```python
from build123d import *

# Parameters (mm, degrees)
SKETCH_1_R               = 67.5
EXTRUDE_1_DEPTH          = 5
SKETCH_2_W               = 6
SKETCH_2_H               = 35
EXTRUDE_2_DEPTH          = 60
FILLET_1_R               = 17.5
SKETCH_3_R               = 16
CUT_EXTRUDE_1_DEPTH      = 5
CHAMFER_1_SIZE           = 1.640243073
CHAMFER_1_SIZE_2         = 0.8
SKETCH_4_R               = 15
CUT_EXTRUDE_2_DEPTH      = 121.188675061
SKETCH_6_W               = 2
SKETCH_6_H               = 6
CUT_EXTRUDE_3_DEPTH      = 121.817372977
SKETCH_8_R               = 1.6
CUT_EXTRUDE_5_DEPTH      = 6
CUT_EXTRUDE_START        = -2
CUT_EXTRUDE_8_DEPTH      = 2.2
SKETCH_11_W              = 25
SKETCH_11_H              = 10.5
EXTRUDE_4_DEPTH          = 7.3
EXTRUDE_5_DEPTH          = 2
FILLET_3_R               = 1
EXTRUDE_6_DEPTH          = 5
SKETCH_14_R              = 1.15
CUT_EXTRUDE_10_DEPTH     = 127.019830237
FILLET_2_R               = 0.5
SKETCH_15_R              = 2
CUT_EXTRUDE_11_DEPTH     = 10
SKETCH_16_W              = 56.328401117
SKETCH_16_H              = 65
CUT_EXTRUDE_12_DEPTH     = 2
SKETCH_17_W              = 112.249721604
SKETCH_17_H              = 30
CUT_EXTRUDE_13_DEPTH     = 113.749722891
SKETCH2_W                = 0.5
SKETCH2_H                = 16.5
BOSS_EXTRUDE1_DEPTH      = 6
BOSS_EXTRUDE2_DEPTH      = 0.5
BOSS_EXTRUDE2_DEPTH_BACK = 3
FILLET1_R                = 1
BOSS_EXTRUDE3_DEPTH      = 0.5
SKETCH5_OUTSIDE_W        = 173.686
SKETCH5_OUTSIDE_H        = 144.186
SKETCH5_OUTSIDE_R        = 67.5
CUT_EXTRUDE1_DEPTH       = 10
SKETCH6_W                = 2.105553893
SKETCH6_H                = 9.3
BOSS_EXTRUDE4_DEPTH      = 3
FILLET2_R                = 1
CUT_EXTRUDE2_START       = -2
CUT_EXTRUDE2_DEPTH       = 2


# Some blends are built 0.0001 mm under size
with BuildPart() as part:
    # 스케치1 → 보스-돌출1 (new body)
    with BuildSketch(Plane(origin=(0, 0, 0), x_dir=(1, 0, 0), z_dir=(0, 1, 0))):
        with Locations(Location((0, 0, 0), (0, 0, 270))):
            Circle(SKETCH_1_R)
    extrude(amount=EXTRUDE_1_DEPTH)

    # 스케치2 → 보스-돌출2 (add)
    with BuildSketch(Plane(origin=(0, 5, 0), x_dir=(1, 0, 0), z_dir=(0, 1, 0))):
        with Locations((5.76, -20)):
            Rectangle(SKETCH_2_W, SKETCH_2_H)
    extrude(amount=EXTRUDE_2_DEPTH)

    # 필렛1
    fillet_1_edges = [part.edges().sort_by_distance(p)[0] for p in [
        (5.76, 65, 2.5),
        (5.76, 65, 37.5),
    ]]
    fillet(fillet_1_edges, radius=FILLET_1_R - 0.0001)  # a hair under: the kernel refuses the full size

    # 스케치3 → 컷-돌출1 (cut)
    with BuildSketch(Plane.ZY.offset(-2.76)):
        with Locations((20, 47.5)):
            Circle(SKETCH_3_R)
    extrude(amount=-CUT_EXTRUDE_1_DEPTH, mode=Mode.SUBTRACT)

    # 모따기1
    # the kernel refuses this chamfer: 1.640243073, 0.8 mm, written as the material it takes off along each edge
    with BuildSketch(Plane(origin=(2.76, 47.5, 20), x_dir=(0, 0, 1), z_dir=(0, -1, 0))) as chamfer_1_piece_1:
        Polygon((16 + CHAMFER_1_SIZE, 0), (16, -CHAMFER_1_SIZE_2), (16, 0), align=None)
    revolve(axis=Axis((2.76, 47.5, 20), (-1, 0, 0)), mode=Mode.SUBTRACT)

    # 스케치4 → 컷-돌출2 (cut, through all)
    with BuildSketch(Plane.ZY.offset(-7.76)):
        with Locations((20, 47.5)):
            Circle(SKETCH_4_R)
    extrude(amount=-CUT_EXTRUDE_2_DEPTH, mode=Mode.SUBTRACT)

    # 스케치6 → 컷-돌출3 (cut, through all)
    with BuildSketch(Plane(origin=(8.76, 0, 0), x_dir=(0, 0, -1), z_dir=(1, 0, 0))):
        with Locations((-3.5, 24.5)):
            Rectangle(SKETCH_6_W, SKETCH_6_H)
    extrude(amount=-CUT_EXTRUDE_3_DEPTH, mode=Mode.SUBTRACT)

    # 스케치8 → 컷-돌출5 (cut)
    with BuildSketch(Plane(origin=(0, 0, 4.5), x_dir=(-1, 0, 0), z_dir=(0, 0, -1))):
        with Locations((-5.76, 24.5)):
            Circle(SKETCH_8_R)
    extrude(amount=-CUT_EXTRUDE_5_DEPTH, mode=Mode.SUBTRACT)

    # 스케치9 → 컷-돌출8 (cut)
    with BuildSketch(Plane(origin=(0, 0, 4.5), x_dir=(-1, 0, 0), z_dir=(0, 0, -1)).offset(CUT_EXTRUDE_START)):
        Polygon((-4.316624327, 27), (-7.203375673, 27), (-8.646751346, 24.5), (-7.203375673, 22), (-4.316624327, 22), (-2.76, 22), (-2.76, 27), align=None)
    extrude(amount=-CUT_EXTRUDE_8_DEPTH, mode=Mode.SUBTRACT)

    # 스케치11 → 보스-돌출4 (add)
    with BuildSketch(Plane(origin=(0, 5, 0), x_dir=(1, 0, 0), z_dir=(0, 1, 0))):
        with Locations((24.26, -7.75)):
            Rectangle(SKETCH_11_W, SKETCH_11_H)
        with Locations((24.26, -32.25)):
            Rectangle(SKETCH_11_W, SKETCH_11_H)
    extrude(amount=EXTRUDE_4_DEPTH)

    # 스케치12 → 보스-돌출5 (add)
    with BuildSketch(Plane(origin=(0, 12.3, 0), x_dir=(1, 0, 0), z_dir=(0, 1, 0))):
        Polygon((16.76, -32.5), (36.76, -32.5), (36.76, -37.5), (11.76, -37.5), (11.76, -27), (16.76, -27), align=None)
        Polygon((11.76, -2.5), (36.76, -2.5), (36.76, -7.5), (16.76, -7.5), (16.76, -13), (11.76, -13), align=None)
    extrude(amount=EXTRUDE_5_DEPTH)

    # 필렛3
    fillet_3_edges = [part.edges().sort_by_distance(p)[0] for p in [
        (36.76, 9.65, 2.5),
        (36.76, 9.65, 37.5),
        (36.76, 8.65, 27),
        (36.76, 8.65, 13),
    ]]
    fillet(fillet_3_edges, radius=FILLET_3_R)

    # 스케치13 → 보스-돌출6 (add)
    with BuildSketch(Plane(origin=(16.76, 0, 0), x_dir=(0, 0, -1), z_dir=(1, 0, 0))):
        with BuildLine():
            Line((-27, 14.3), (-37.5, 14.3))
            Line((-37.5, 14.3), (-37.5, 44.3))
            Line((-37.5, 44.3), (-30.524257694, 44.3))
            ThreePointArc((-30.524257694, 44.3), (-29.151964364, 41.397414624), (-27, 39.014718626))
            Line((-27, 39.014718626), (-27, 14.3))
        make_face()
        with BuildLine():
            Line((-13, 14.3), (-2.5, 14.3))
            Line((-2.5, 14.3), (-2.5, 44.3))
            Line((-2.5, 44.3), (-9.475742306, 44.3))
            ThreePointArc((-9.475742306, 44.3), (-10.848035636, 41.397414624), (-13, 39.014718626))
            Line((-13, 39.014718626), (-13, 14.3))
        make_face()
    extrude(amount=-EXTRUDE_6_DEPTH)

    # 스케치14 → 컷-돌출10 (cut, through all)
    with BuildSketch(Plane(origin=(16.76, 0, 0), x_dir=(0, 0, -1), z_dir=(1, 0, 0))):
        with Locations((-30.25, 18.3)):
            Circle(SKETCH_14_R)
        with Locations((-9.75, 18.3)):
            Circle(SKETCH_14_R)
        with Locations((-9.75, 38.8)):
            Circle(SKETCH_14_R)
        with Locations((-30.25, 38.8)):
            Circle(SKETCH_14_R)
    extrude(amount=-CUT_EXTRUDE_10_DEPTH, mode=Mode.SUBTRACT)

    # 필렛2
    fillet_2_edges = [part.edges().sort_by_distance(p)[0] for p in [
        (26.26, 12.3, 13),
        (16.76, 25.657359313, 13),
        (26.76, 12.3, 7.5),
        (36.76, 13.3, 7.5),
        (36.76, 12.3, 30.25),
        (16.76, 25.657359313, 27),
        (26.76, 12.3, 32.5),
        (36.76, 13.3, 32.5),
        (26.26, 12.3, 27),
        (36.467106781, 12.3, 27.292893219),
        (36.76, 12.3, 9.75),
        (36.467106781, 12.3, 12.707106781),
    ]]
    fillet(fillet_2_edges, radius=FILLET_2_R)

    # 스케치15 → 컷-돌출11 (cut)
    with BuildSketch(Plane.ZY.offset(-2.76)):
        with Locations((9.75, 38.8)):
            Circle(SKETCH_15_R)
        with Locations((30.25, 38.8)):
            Circle(SKETCH_15_R)
        with Locations((9.75, 18.3)):
            Circle(SKETCH_15_R)
        with Locations((30.25, 18.3)):
            Circle(SKETCH_15_R)
    extrude(amount=-CUT_EXTRUDE_11_DEPTH, mode=Mode.SUBTRACT)

    # 스케치16 → 컷-돌출12 (cut)
    with BuildSketch(Plane(origin=(0, 5, 0), x_dir=(1, 0, 0), z_dir=(0, 1, 0))):
        with Locations((-39.335799442, -35)):
            Rectangle(SKETCH_16_W, SKETCH_16_H)
    extrude(amount=-CUT_EXTRUDE_12_DEPTH, mode=Mode.SUBTRACT)

    # 스케치17 → 컷-돌출13 (cut, through all)
    with BuildSketch(Plane(origin=(0, 5, 0), x_dir=(1, 0, 0), z_dir=(0, 1, 0))):
        with Locations((0, -52.5)):
            Rectangle(SKETCH_17_W, SKETCH_17_H)
    extrude(amount=-CUT_EXTRUDE_13_DEPTH, mode=Mode.SUBTRACT)

    # Sketch2 → Boss-Extrude1 (add)
    with BuildSketch(Plane.ZY.offset(-2.76)):
        with BuildLine():
            Line((2, 27.5), (2, 47.5))
            ThreePointArc((2, 47.5), (20, 65.5), (38, 47.5))
            Line((38, 47.5), (38, 5))
            Line((38, 5), (37.5, 5))
            Line((37.5, 5), (37.5, 45.280050522))
            Line((37.5, 45.280050522), (37.5, 47.5))
            ThreePointArc((37.5, 47.5), (32.374368671, 59.874368671), (20, 65))
            ThreePointArc((20, 65), (7.625631329, 59.874368671), (2.5, 47.5))
            Line((2.5, 47.5), (2.5, 45.280050522))
            Line((2.5, 45.280050522), (2.5, 27.5))
            Line((2.5, 27.5), (2, 27.5))
        make_face()
        with Locations((2.25, 13.25)):
            Rectangle(SKETCH2_W, SKETCH2_H)
    extrude(amount=-BOSS_EXTRUDE1_DEPTH)

    # Sketch3 → Boss-Extrude2 (add, two sides: drawn at the far end of the back side and taken through both)
    with BuildSketch(Plane(origin=(0, 0, 2.5), x_dir=(-1, 0, 0), z_dir=(0, 0, -1)).offset(-BOSS_EXTRUDE2_DEPTH_BACK)):
        Polygon((-36.76, 5), (-36.76, 14.3), (-16.76, 14.3), (-16.76, 44.3), (-11.76, 44.3), (-11.76, 5), align=None)
    extrude(amount=BOSS_EXTRUDE2_DEPTH + BOSS_EXTRUDE2_DEPTH_BACK)

    # Fillet1
    fillet1_edges = [part.edges().sort_by_distance(p)[0] for p in [
        (36.76, 9.65, 2),
    ]]
    fillet(fillet1_edges, radius=FILLET1_R)

    # Sketch4 → Boss-Extrude3 (add)
    with BuildSketch(Plane.XY.offset(37.5)):
        Polygon((11.76, 5), (8.76, 5), (2.76, 5), (-11.171598883, 5), (-11.171598883, 3), (-56.124860802, 3), (-56.124860802, 0), (56.124860802, 0), (56.124860802, 5), (35.76, 5), (35.76, 14.3), (16.76, 14.3), (16.76, 44.3), (11.76, 44.3), align=None)
    extrude(amount=BOSS_EXTRUDE3_DEPTH)

    # Sketch5 outside → Cut-Extrude1 (cut)
    with BuildSketch(Plane.XZ):
        with Locations((0, -14.75)):
            Rectangle(SKETCH5_OUTSIDE_W, SKETCH5_OUTSIDE_H)
        Circle(SKETCH5_OUTSIDE_R, mode=Mode.SUBTRACT)
    extrude(amount=-CUT_EXTRUDE1_DEPTH, mode=Mode.SUBTRACT)

    # Sketch6 → Boss-Extrude4 (add)
    with BuildSketch(Plane.XY.offset(38)):
        with Locations((35.707223054, 9.65)):
            Rectangle(SKETCH6_W, SKETCH6_H)
    extrude(amount=-BOSS_EXTRUDE4_DEPTH)

    # Fillet2
    fillet2_edges = [part.edges().sort_by_distance(p)[0] for p in [
        (36.76, 9.65, 38),
    ]]
    fillet(fillet2_edges, radius=FILLET2_R)

    # Sketch7 → Cut-Extrude2 (cut)
    with BuildSketch(Plane(origin=(0, 5, 0), x_dir=(1, 0, 0), z_dir=(0, 1, 0)).offset(CUT_EXTRUDE2_START)):
        with BuildLine():
            Line((-11.171598883, -2), (-11.171598883, -2.5))
            Line((-11.171598883, -2.5), (-67.453687816, -2.5))
            ThreePointArc((-67.453687816, -2.5), (-67.462489062, -2.250015449), (-67.470363864, -2))
            Line((-67.470363864, -2), (-11.171598883, -2))
        make_face()
    extrude(amount=CUT_EXTRUDE2_DEPTH, mode=Mode.SUBTRACT)


solid = part.part
```
CAD build for the part. Positions are in the model's coordinates, mm. A direction names the side the tool comes from. Coordinates: 2 decimals unless noted, no trailing zeros. Order: outer loops, then holes, each group sorted by start corner. A loop starts at its lowest first (then second) coordinate and runs counter-clockwise, first axis right, second up. Notation, with made-up numbers: M 41,60.25 L 61,60.25 A20 cw 61,91.25 Z; hole C 54.5,30 d2. An arc over 180 degrees is marked long. Write each question's results on one line, items separated by ' | '. Start each with the question number.
Q1. Pull direction Y, two halves, no side cores. Call faces 4 (the cylindrical face through (12.253, 18.901, 32.158)), 5 (the flat face through (-1, 0, -15)), 6 (the flat face through (36.76, 10, 8)): +Y half, -Y half, draft (parallel to the pull), parting line (faces both ways), or undercut.
Q2. Cut at D-D (z = -43). List the corners of the cut face in (x, y).
Q3. Cut at A-A (x = 23). List the corners of the cut face in (y, z), then the cut area to 3 significant figures.
Q4. Drill centre lines: probe 1 along Y at (x, z) = (12, 9); probe 2 along Z at (x, y) = (14, 38); probe 3 along Y at (x, z) = (0, -8). Where is each one in solid material? Low to high. Write a range as from..to.
Q5. Flat gauge pins, fed straight in: P1, Ø3, axis at y = 18.3, z = 9.75, coming from the -X side; P2, Ø4.5, axis at y = 18.3, z = 9.75, coming from the -X side; P3, Ø5.5, axis at y = 29, z = 7, coming from the +X side. Where does each tip first touch, or does it go through?
Q6. Cut at B-B (z = 0). List the corners of the cut face in (x, y), then the cut area to 3 significant figures.
Q7. Which spindle directions (+Z, -Z, +X, -X, +Y, -Y) get a long thin tool onto all of the face, cutting with end or side? Do faces 1 (the flat face through (6, 13, 2)), 2 (the flat face through (16, 15, 27)), 3 (the cylindrical face through (8.253, 62.493, 20.459)). Say none if no direction does.
Q8. Cut at C-C (x = -19.5). List the corners of the cut face in (y, z), then the cut area to 3 significant figures.
Found:
1) face 4: undercut | face 5: -Y half | face 6: draft
2) outline: M -52.03,0 L 52.03,0 L 52.03,5 L -52.03,5 Z
3) outline: M 0,-63.46 L 5,-63.46 L 5,2 L 14.3,2 L 14.3,7.5 L 12.8,7.5 A0.5 cw 12.3,8 L 12.3,12.5 A0.5 ccw 11.8,13 L 5,13 L 5,27 L 11.8,27 A0.5 ccw 12.3,27.5 L 12.3,32 A0.5 cw 12.8,32.5 L 14.3,32.5 L 14.3,38 L 0,38 Z | area: 690 mm²
4) probe 1: 0..16.45, 20.15..36.95, 40.65..44.3 | probe 2: 2..8.92, 10.58..13, 27..29.42, 31.08..38 | probe 3: 0..5
5) P1: x = 12.76 | P2: x = 2.76 | P3: x = 16.76
6) outline: M -67.5,0 L 67.5,0 L 67.5,5 L -67.5,5 Z | area: 675 mm²
7) face 1: -Z, +X, -X, +Y | face 2: +X, +Y | face 3: -X
8) outline: M 0,-64.62 L 5,-64.62 L 5,2 L 3,2 L 3,38 L 0,38 Z | area: 441 mm²
